from build123d import *

# Parameters (mm, degrees)
F0_W     = 84
F0_H     = 40
F0_R     = 1.45
F1_DEPTH = 1
F2_DEPTH = 12
F3_DEPTH = 14
F4_W     = 11
F4_H     = 12
F5_DEPTH = 25
F7_DEPTH = 1


with BuildPart() as f1:
    # F0 (on Top) → F1 (new body)
    with BuildSketch(Plane.XY):
        with Locations((-0.4375013113, -5.1794923829)):
            Rectangle(F0_W, F0_H)
        Polygon((-40.6875013113, 8.0205076171), (-40.6875013113, 13.0705076171), (-35.6375013113, 13.0705076171), (34.7624986887, 13.0705076171), (39.8124986887, 13.0705076171), (39.8124986887, 8.0205076171), (39.8124986887, -18.3794923829), (39.8124986887, -23.4294923829), (34.7624986887, -23.4294923829), (-35.6375013113, -23.4294923829), (-40.6875013113, -23.4294923829), (-40.6875013113, -18.3794923829), align=None, mode=Mode.SUBTRACT)
        with BuildLine():
            Line((34.7624986887, 13.0705076171), (-35.6375013113, 13.0705076171))
            Line((-35.6375013113, 13.0705076171), (-35.6375013113, 10.5205076171))
            ThreePointArc((-35.6375013113, 10.5205076171), (-36.3697343583, 8.7527406642), (-38.1375013113, 8.0205076171))
            Line((-38.1375013113, 8.0205076171), (-40.6875013113, 8.0205076171))
            Line((-40.6875013113, 8.0205076171), (-40.6875013113, -18.3794923829))
            Line((-40.6875013113, -18.3794923829), (-38.1375013113, -18.3794923829))
            ThreePointArc((-38.1375013113, -18.3794923829), (-36.3697343583, -19.1117254299), (-35.6375013113, -20.8794923829))
            Line((-35.6375013113, -20.8794923829), (-35.6375013113, -23.4294923829))
            Line((-35.6375013113, -23.4294923829), (34.7624986887, -23.4294923829))
            Line((34.7624986887, -23.4294923829), (34.7624986887, -20.8794923829))
            ThreePointArc((34.7624986887, -20.8794923829), (35.4947317357, -19.1117254299), (37.2624986887, -18.3794923829))
            Line((37.2624986887, -18.3794923829), (39.8124986887, -18.3794923829))
            Line((39.8124986887, -18.3794923829), (39.8124986887, 8.0205076171))
            Line((39.8124986887, 8.0205076171), (37.2624986887, 8.0205076171))
            ThreePointArc((37.2624986887, 8.0205076171), (35.4947317357, 8.7527406642), (34.7624986887, 10.5205076171))
            Line((34.7624986887, 10.5205076171), (34.7624986887, 13.0705076171))
        make_face()
        with BuildLine():
            Line((39.8124986887, -23.4294923829), (39.8124986887, -18.3794923829))
            Line((39.8124986887, -18.3794923829), (37.2624986887, -18.3794923829))
            ThreePointArc((37.2624986887, -18.3794923829), (35.4947317357, -19.1117254299), (34.7624986887, -20.8794923829))
            Line((34.7624986887, -20.8794923829), (34.7624986887, -23.4294923829))
            Line((34.7624986887, -23.4294923829), (39.8124986887, -23.4294923829))
        make_face()
        with Locations((37.2624986887, -20.8794923829)):
            Circle(F0_R, mode=Mode.SUBTRACT)
        with BuildLine():
            Line((39.8124986887, 13.0705076171), (34.7624986887, 13.0705076171))
            Line((34.7624986887, 13.0705076171), (34.7624986887, 10.5205076171))
            ThreePointArc((34.7624986887, 10.5205076171), (35.4947317357, 8.7527406642), (37.2624986887, 8.0205076171))
            Line((37.2624986887, 8.0205076171), (39.8124986887, 8.0205076171))
            Line((39.8124986887, 8.0205076171), (39.8124986887, 13.0705076171))
        make_face()
        with Locations((37.2624986887, 10.5205076171)):
            Circle(F0_R, mode=Mode.SUBTRACT)
        with BuildLine():
            Line((-38.1375013113, -18.3794923829), (-40.6875013113, -18.3794923829))
            Line((-40.6875013113, -18.3794923829), (-40.6875013113, -23.4294923829))
            Line((-40.6875013113, -23.4294923829), (-35.6375013113, -23.4294923829))
            Line((-35.6375013113, -23.4294923829), (-35.6375013113, -20.8794923829))
            ThreePointArc((-35.6375013113, -20.8794923829), (-36.3697343583, -19.1117254299), (-38.1375013113, -18.3794923829))
        make_face()
        with Locations((-38.1375013113, -20.8794923829)):
            Circle(F0_R, mode=Mode.SUBTRACT)
        with BuildLine():
            Line((-35.6375013113, 13.0705076171), (-40.6875013113, 13.0705076171))
            Line((-40.6875013113, 13.0705076171), (-40.6875013113, 8.0205076171))
            Line((-40.6875013113, 8.0205076171), (-38.1375013113, 8.0205076171))
            ThreePointArc((-38.1375013113, 8.0205076171), (-36.3697343583, 8.7527406642), (-35.6375013113, 10.5205076171))
            Line((-35.6375013113, 10.5205076171), (-35.6375013113, 13.0705076171))
        make_face()
        with Locations((-38.1375013113, 10.5205076171)):
            Circle(F0_R, mode=Mode.SUBTRACT)
        with Locations((37.2624986887, 10.5205076171)):
            Circle(F0_R)
        with Locations((-38.1375013113, 10.5205076171)):
            Circle(F0_R)
        with Locations((37.2624986887, -20.8794923829)):
            Circle(F0_R)
        with Locations((-38.1375013113, -20.8794923829)):
            Circle(F0_R)
    extrude(amount=F1_DEPTH)

    # F0 (on Top) → F2 (join)
    with BuildSketch(Plane.XY):
        with BuildLine():
            Line((-35.6375013113, 13.0705076171), (-40.6875013113, 13.0705076171))
            Line((-40.6875013113, 13.0705076171), (-40.6875013113, 8.0205076171))
            Line((-40.6875013113, 8.0205076171), (-38.1375013113, 8.0205076171))
            ThreePointArc((-38.1375013113, 8.0205076171), (-36.3697343583, 8.7527406642), (-35.6375013113, 10.5205076171))
            Line((-35.6375013113, 10.5205076171), (-35.6375013113, 13.0705076171))
        make_face()
        with Locations((-38.1375013113, 10.5205076171)):
            Circle(F0_R, mode=Mode.SUBTRACT)
        with BuildLine():
            Line((39.8124986887, 13.0705076171), (34.7624986887, 13.0705076171))
            Line((34.7624986887, 13.0705076171), (34.7624986887, 10.5205076171))
            ThreePointArc((34.7624986887, 10.5205076171), (35.4947317357, 8.7527406642), (37.2624986887, 8.0205076171))
            Line((37.2624986887, 8.0205076171), (39.8124986887, 8.0205076171))
            Line((39.8124986887, 8.0205076171), (39.8124986887, 13.0705076171))
        make_face()
        with Locations((37.2624986887, 10.5205076171)):
            Circle(F0_R, mode=Mode.SUBTRACT)
        with BuildLine():
            Line((39.8124986887, -23.4294923829), (39.8124986887, -18.3794923829))
            Line((39.8124986887, -18.3794923829), (37.2624986887, -18.3794923829))
            ThreePointArc((37.2624986887, -18.3794923829), (35.4947317357, -19.1117254299), (34.7624986887, -20.8794923829))
            Line((34.7624986887, -20.8794923829), (34.7624986887, -23.4294923829))
            Line((34.7624986887, -23.4294923829), (39.8124986887, -23.4294923829))
        make_face()
        with Locations((37.2624986887, -20.8794923829)):
            Circle(F0_R, mode=Mode.SUBTRACT)
        with BuildLine():
            Line((-38.1375013113, -18.3794923829), (-40.6875013113, -18.3794923829))
            Line((-40.6875013113, -18.3794923829), (-40.6875013113, -23.4294923829))
            Line((-40.6875013113, -23.4294923829), (-35.6375013113, -23.4294923829))
            Line((-35.6375013113, -23.4294923829), (-35.6375013113, -20.8794923829))
            ThreePointArc((-35.6375013113, -20.8794923829), (-36.3697343583, -19.1117254299), (-38.1375013113, -18.3794923829))
        make_face()
        with Locations((-38.1375013113, -20.8794923829)):
            Circle(F0_R, mode=Mode.SUBTRACT)
    extrude(amount=F2_DEPTH)

    # F0 (on Top) → F3 (join)
    with BuildSketch(Plane.XY):
        with Locations((-0.4375013113, -5.1794923829)):
            Rectangle(F0_W, F0_H)
        Polygon((-40.6875013113, 8.0205076171), (-40.6875013113, 13.0705076171), (-35.6375013113, 13.0705076171), (34.7624986887, 13.0705076171), (39.8124986887, 13.0705076171), (39.8124986887, 8.0205076171), (39.8124986887, -18.3794923829), (39.8124986887, -23.4294923829), (34.7624986887, -23.4294923829), (-35.6375013113, -23.4294923829), (-40.6875013113, -23.4294923829), (-40.6875013113, -18.3794923829), align=None, mode=Mode.SUBTRACT)
    extrude(amount=F3_DEPTH)

    # F4 (on face) → F5 (cut)
    with BuildSketch(Plane(origin=(-42.4375013113, 0, 0), x_dir=(0, -1, 0), z_dir=(-1, 0, 0))):
        with Locations((-2.5705076171, 8)):
            Rectangle(F4_W, F4_H)
    extrude(amount=-F5_DEPTH, mode=Mode.SUBTRACT)

    # F6 (on face) → F7 (cut)
    with BuildSketch(Plane.XY.offset(14)):
        Polygon((40.8124986887, 14.0705076171), (-41.4375013113, 14.0705076171), (-41.4375013113, 8.0705076171), (-40.6875013113, 8.0705076171), (-40.6875013113, 13.0705076171), (39.8124986887, 13.0705076171), (39.8124986887, -23.4294923829), (-40.6875013113, -23.4294923829), (-40.6875013113, -2.9294923829), (-41.4375013113, -2.9294923829), (-41.4375013113, -24.4294923829), (40.8124986887, -24.4294923829), align=None)
    extrude(amount=-F7_DEPTH, mode=Mode.SUBTRACT)


solid = f1.part
Work out the finished part from the listing and answer in its coordinate system (mm). A direction names the side the tool comes from. Give positions to 0.01 mm unless a question says otherwise; leave off trailing zeros. Order: outer loops, then holes, each group sorted by start corner. A loop starts at its lowest first (then second) coordinate and runs counter-clockwise, first axis right, second up. Notation, with made-up numbers: (-1, 50) -> (16, 50) arc R23 ccw to (16, 79) -> close; hole circle Ø9 at (42.25, 70). An arc over 180 degrees is marked (long way). Answer as a JSON object with one key per item and string values. Group by question number.
1. Section B-B on z = 7.5 is taken. Determine the outline of the cut face in (x, y).
2. Section A-A on y = -15 is taken. Determine the outline of the cut face in (x, z).
3. Section C-C on x = 13 is taken. Determine the outline of the cut face in (y, z), plus the area to 3 significant figures.
4. A tool of negligible diameter and unlimited length cuts with its end or side. For faces 4 (the flat face through (37, 11, 1)), 5 (the flat face through (-1, -5, 0)), 6 (the flat face through (-42, 3, 2)), from which of +Z, -Z, +X, -X, +Y, -Y can it reach the whole face along a straight path? Write none if from no direction.
5. Section D-D on y = 0.5 is taken. Determine the outline of the cut face in (x, z), plus the area to 4 significant figures.
6. The mould has two halves that part along Y. Classify faces 1 (the flat face through (-35.638, 12, 6)), 2 (the flat face through (-42.438, -10, 7)), 3 (the flat face through (-1, 14.821, 7)): released by +Y, released by -Y, zero draft, split by the parting line, or undercut.
7. Consider line 1 along X through (y, z) = (10.5, 6.75); line 2 along X through (y, z) = (-18, 12.75); line 3 along Y through (x, z) = (-24, 6.5). Determine where each line is inside the solid, lowest interval first. Write a range as [from, to].
8. Flat-ended cylindrical pins translate along their axes: pin 1 Ø4 at (x, y) = (-38.14, -20.88) entering from +Z; pin 2 Ø1.7 at (x, y) = (37.26, -20.88) entering from +Z; pin 3 Ø4 at (x, y) = (-37.5, -22) entering from +Z. Find the tip coordinate at first contact, or state that the pin passes through.
Result sheet:
{
 "1": {"outline": "(-42.44, -25.18) -> (41.56, -25.18) -> (41.56, 14.82) -> (-42.44, 14.82) -> (-42.44, 8.07) -> (-37.64, 8.07) arc R2.5 ccw to (-35.64, 10.52) -> (-35.64, 13.07) -> (34.76, 13.07) -> (34.76, 10.52) arc R2.5 ccw to (37.26, 8.02) -> (39.81, 8.02) -> (39.81, -18.38) -> (37.26, -18.38) arc R2.5 ccw to (34.76, -20.88) -> (34.76, -23.43) -> (-35.64, -23.43) -> (-35.64, -20.88) arc R2.5 ccw to (-38.14, -18.38) -> (-40.69, -18.38) -> (-40.69, -2.93) -> (-42.44, -2.93) -> close; hole circle Ø2.9 at (-38.14, -20.88); hole circle Ø2.9 at (-38.14, 10.52); hole circle Ø2.9 at (37.26, -20.88); hole circle Ø2.9 at (37.26, 10.52)"},
 "2": {"outline": "(-42.44, 0) -> (41.56, 0) -> (41.56, 14) -> (40.81, 14) -> (40.81, 13) -> (39.81, 13) -> (39.81, 1) -> (-40.69, 1) -> (-40.69, 13) -> (-41.44, 13) -> (-41.44, 14) -> (-42.44, 14) -> close"},
 "3": {"outline": "(-25.18, 0) -> (14.82, 0) -> (14.82, 14) -> (14.07, 14) -> (14.07, 13) -> (13.07, 13) -> (13.07, 1) -> (-23.43, 1) -> (-23.43, 13) -> (-24.43, 13) -> (-24.43, 14) -> (-25.18, 14) -> close", "area": "83.5 mm^2"},
 "4": {"face 4": "+Z", "face 5": "-Z, +X, -X, +Y, -Y", "face 6": "+Z, -X"},
 "5": {"outline": "(-42.44, 0) -> (41.56, 0) -> (41.56, 14) -> (40.81, 14) -> (40.81, 13) -> (39.81, 13) -> (39.81, 1) -> (-40.69, 1) -> (-40.69, 2) -> (-42.44, 2) -> close", "area": "107.5 mm^2"},
 "6": {"face 1": "undercut", "face 2": "zero draft", "face 3": "released by +Y"},
 "7": {"line 1": "x = [-42.44, -39.59], [-36.69, -35.64], [34.76, 35.81], [38.71, 41.56]", "line 2": "x = [-42.44, -40.69], [39.81, 41.56]", "line 3": "y = [-25.18, -23.43], [13.07, 14.82]"},
 "8": {"pin 1": "stops at z = 12", "pin 2": "stops at z = 1", "pin 3": "stops at z = 13"}
}
